Verification items for the finished model (mm, model axes). A direction names the side the tool comes from. Round coordinates to 2 decimals unless told otherwise and drop trailing zeros. Write each loop counter-clockwise with the first axis right and the second up, starting at its lowest first coordinate (ties: lowest second). Pieces come first, ordered by that corner, then holes. Notation, with made-up numbers: (-7, 60.5) -> (4, 60.5) arc R13 ccw to (4, 73.5) -> close; hole circle Ø9 at (64.25, -11). An arc over 180 degrees is marked (long way). Answer as a JSON object with one key per item and string values. Group by question number.
(1) Sectioned sample at D-D on x = 100. Count the separate pieces of the cut face and the enclosed holes in it, and give its area (3 significant figures).
(2) Draft check along X on faces 4 (the face through (128, 4, 4)), 5 (the face through (43.02, 19.31, 1.48)), 6 (the face through (70.94, 79.14, 0.9)), 7 (the face through (101.15, 67.78, 1.48)). Enter one of: released by +X, released by -X, zero draft, split by the parting line, or undercut.
(3) Gauge pin test, flat ends, axial feed: pin 1 Ø2 at (x, z) = (42.5, 3.5) entering from +Y; pin 2 Ø1 at (x, z) = (58.5, 4.5) entering from -Y; pin 3 Ø1.5 at (x, z) = (80.5, 4) entering from +Y; pin 4 Ø2.5 at (x, z) = (4.5, 4.5) entering from -Y. Record the tip position at first contact, or that the pin passes through.
(4) Set-up check for faces 1 (the face through (135, 12, 4)), 2 (the face through (69, 5.5, 4)), 3 (the face through (6, 40, 4)): record each of +Z, -Z, +X, -X, +Y, -Y from which the full face is reachable in a straight line by a thin tool's end or side.
(5) Sectioned sample at C-C on z = 4.5. Record the cut outline in (x, y), and give its area (3 significant figures).
(6) Scan lines: L1, parallel to Y at x = 63, z = 5.05; L2, parallel to Y at x = 40, z = 1.1; L3, parallel to Y at x = 40, z = 0.9. Record each from-to range of solid material in increasing order. Write a range as from..to.
```python
from build123d import *

# Parameters (mm, degrees)
F0_W     = 116
F0_H     = 2.5
F1_DEPTH = 6
F0_W_2   = 3
F0_H_2   = 56
F0_W_3   = 140
F0_H_3   = 80
F0_R     = 1.5
F0_R_2   = 2.5
F0_R_3   = 34
F2_DEPTH = 3
F3_R     = 2.99999


# Not quite as in the source:
# - a fillet or chamfer is up to 0.001 mm smaller than in the source, because OpenCascade refuses the exact size


with BuildPart() as f1:
    # F0 (on Top) → F1 (new body)
    with BuildSketch(Plane.XY):
        with Locations((70, 75.75)):
            Rectangle(F0_W, F0_H)
    extrude(amount=F1_DEPTH)



with BuildPart() as f1b:
    # F0 (on Top) → F1, piece 2 (new body)
    with BuildSketch(Plane.XY):
        with Locations((70, 4.25)):
            Rectangle(F0_W, F0_H)
    extrude(amount=F1_DEPTH)


with BuildPart() as f1c:
    # F0 (on Top) → F1, piece 3 (new body)
    with BuildSketch(Plane.XY):
        with Locations((4.5, 40)):
            Rectangle(F0_W_2, F0_H_2)
    extrude(amount=F1_DEPTH)


with BuildPart() as f1d:
    # F0 (on Top) → F1, piece 4 (new body)
    with BuildSketch(Plane.XY):
        with Locations((135.5, 40)):
            Rectangle(F0_W_2, F0_H_2)
    extrude(amount=F1_DEPTH)


with BuildPart() as f1_1:
    add(f1.part)

    add(f1b.part)  # F2 merges F1b

    add(f1c.part)  # F2 merges F1c

    add(f1d.part)  # F2 merges F1d
    # F0 (on Top) → F2 (join)
    with BuildSketch(Plane.XY):
        with Locations((70, 40)):
            Rectangle(F0_W_3, F0_H_3)
        with Locations((5.5, 5.5)):
            Circle(F0_R, mode=Mode.SUBTRACT)
        with Locations((40, 10)):
            Circle(F0_R_2, mode=Mode.SUBTRACT)
        with Locations((70, 4.25)):
            Rectangle(F0_W, F0_H, mode=Mode.SUBTRACT)
        with Locations((100, 10)):
            Circle(F0_R_2, mode=Mode.SUBTRACT)
        with Locations((134.5, 5.5)):
            Circle(F0_R, mode=Mode.SUBTRACT)
        with Locations((4.5, 40)):
            Rectangle(F0_W_2, F0_H_2, mode=Mode.SUBTRACT)
        with Locations((5.5, 74.5)):
            Circle(F0_R, mode=Mode.SUBTRACT)
        with Locations((40, 70)):
            Circle(F0_R_2, mode=Mode.SUBTRACT)
        with Locations((70, 40)):
            Circle(F0_R_3, mode=Mode.SUBTRACT)
        with Locations((135.5, 40)):
            Rectangle(F0_W_2, F0_H_2, mode=Mode.SUBTRACT)
        with Locations((70, 75.75)):
            Rectangle(F0_W, F0_H, mode=Mode.SUBTRACT)
        with Locations((100, 70)):
            Circle(F0_R_2, mode=Mode.SUBTRACT)
        with Locations((134.5, 74.5)):
            Circle(F0_R, mode=Mode.SUBTRACT)
    extrude(amount=F2_DEPTH)

    # F3 (radius 3 in the source; OpenCascade refuses exactly that, so slightly less here)
    f3_edges = [f1_1.edges().sort_by_distance(p)[0] for p in [
        (140, 40, 0),
        (140, 80, 1.5),
        (0, 0, 1.5),
        (0, 80, 1.5),
        (140, 0, 1.5),
        (70, 0, 0),
        (70, 80, 0),
        (0, 40, 0),
    ]]
    fillet(f3_edges, radius=F3_R)


solid = f1_1.part
```
Computed values:
{
 "1": {"separate pieces": "4", "enclosed holes": "0", "area": "125 mm2"},
 "2": {"face 4": "released by +X", "face 5": "undercut", "face 6": "zero draft", "face 7": "undercut"},
 "3": {"pin 1": "y = 80", "pin 2": "y = 3", "pin 3": "y = 77", "pin 4": "y = 12"},
 "4": {"face 1": "+Z, +X, -X, -Y", "face 2": "+Z, +X, -X", "face 3": "+Z, +Y, -Y"},
 "5": {"outline": "(3, 12) -> (6, 12) -> (6, 68) -> (3, 68) -> close; (12, 3) -> (128, 3) -> (128, 5.5) -> (12, 5.5) -> close; (12, 74.5) -> (128, 74.5) -> (128, 77) -> (12, 77) -> close; (134, 12) -> (137, 12) -> (137, 68) -> (134, 68) -> close", "area": "916 mm2"},
 "6": {"L1": "3..5.5, 74.5..77", "L2": "0.68..7.5, 12.5..24, 56..67.5, 72.5..79.32", "L3": "0.86..7.5, 12.5..24, 56..67.5, 72.5..79.14"}
}
